Work out the finished part from the listing and answer in its coordinate system (mm). A direction names the side the tool comes from. Give positions to 0.01 mm unless a question says otherwise; leave off trailing zeros. Write each loop counter-clockwise with the first axis right and the second up, starting at its lowest first coordinate (ties: lowest second). Pieces come first, ordered by that corner, then holes. Notation, with made-up numbers: (2.5, 2.5) -> (47.5, 2.5) arc R28 cw to (47.5, 23.5) -> close; hole circle Ø11 at (39, 16.5). An arc over 180 degrees is marked (long way). Use a Markdown table: item, result. Add a question column.
Q1. Each of these flat-tipped pins is pushed along its axis until it touches: pin 1 Ø0.7 at (y, z) = (23, 7) entering from -X; pin 2 Ø10 at (y, z) = (6.5, 17.5) entering from +X; pin 3 Ø11 at (y, z) = (14.5, 14) entering from -X; pin 4 Ø7.5 at (x, z) = (-47, 10) entering from -Y. Where does it stop, or does it pass through?
Q2. Section B-B, the plane z = 18.5 is taken. Give the vertices of the cut face in (x, y), plus the area to 3 significant figures.
Q3. For faces 1 (the face through (-26.678, 12.444, 9.86)), 2 (the face through (-48, 23.8, 10)), 3 (the face through (-27, 25, 10)), determine the directions among +Z, -Z, +X, -X, +Y, -Y from which every point of the face is accessible in a straight line to the end or side of a thin tool.
Q4. Section C-C, the plane x = -37.5 is taken. Give the vertices of the cut face in (y, z).
Q5. For a pull along X with two mould halves and no side action, classify faces 4 (the face through (-4, 16, 10)), 5 (the face through (-22, 10, 20)), 6 (the face through (0, 14, 10)) as pulls with the +X half, pulls with the -X half, needs draft (parallel to the pull), parting line crosses it, or undercut.
Q6. Section D-D, the plane y = 17.5 is taken. Give the vertices of the cut face in (x, z).
Q7. Section A-A, the plane x = -46 is taken. Give the vertices of the cut face in (y, z).
Q8. Consider line 1 (X direction, y = 22.75, z = 16); line 2 (X direction, y = 17, z = 18); line 3 (Y direction, x = -44.5, z = 18.75). Determine where each line is inside the solid, lowest interval first.
from build123d import *

# Parameters (mm, degrees)
PAD_DEPTH = 20


with BuildPart() as part:
    # Sketch → Pad (new body)
    with BuildSketch(Plane.XY):
        Polygon((-40, 22.5), (-4, 22.5), (-4, 8.5), (-50, 16.5), (-55, 14.989843), (0, 3.5), (0, 25), (-55, 25), (-55, 23.8), (-40, 23.8), align=None)
    extrude(amount=PAD_DEPTH)


solid = part.part
Result set:
| question | item | result |
|---|---|---|
| 1 | pin 1 | stops at x = -40 |
| 1 | pin 2 | stops at x = 0 |
| 1 | pin 3 | stops at x = -55 |
| 1 | pin 4 | stops at y = 12.54 |
| 2 | outline | (-55, 14.99) -> (0, 3.5) -> (0, 25) -> (-55, 25) -> (-55, 23.8) -> (-40, 23.8) -> (-40, 22.5) -> (-4, 22.5) -> (-4, 8.5) -> (-50, 16.5) -> close |
| 2 | area | 353 mm2 |
| 3 | face 1 | +Z, -Z |
| 3 | face 2 | +Z, -Z, -X |
| 3 | face 3 | +Z, -Z, +X, -X, +Y |
| 4 | outline | (11.33, 0) -> (14.33, 0) -> (14.33, 20) -> (11.33, 20) -> close; (22.5, 0) -> (25, 0) -> (25, 20) -> (22.5, 20) -> close |
| 5 | face 4 | undercut |
| 5 | face 5 | needs draft |
| 5 | face 6 | pulls with the +X half |
| 6 | outline | (-4, 0) -> (0, 0) -> (0, 20) -> (-4, 20) -> close |
| 7 | outline | (13.11, 0) -> (15.8, 0) -> (15.8, 20) -> (13.11, 20) -> close; (23.8, 0) -> (25, 0) -> (25, 20) -> (23.8, 20) -> close |
| 8 | line 1 | x = -40 to 0 |
| 8 | line 2 | x = -4 to 0 |
| 8 | line 3 | y = 12.8 to 15.54, 23.8 to 25 |
